```python
from build123d import *

# Parameters (mm, degrees)
F1_DEPTH = 8
F2_R     = 2
F3_R     = 3
F4_R     = 2.5
F5_DEPTH = 8.001
F7_DEPTH = 8.001


with BuildPart() as f1:
    # F0 (on Front) → F1 (new body)
    with BuildSketch(Plane.XZ):
        Polygon((-37.1, 0), (-33.1, 0), (-33.1, 9), (-27.1, 9), (-27.1, 13), (0, 13), (0, 19), (-37.1, 19), align=None)
    extrude(amount=F1_DEPTH)

    # F2
    f2_edges = [f1.edges().sort_by_distance(p)[0] for p in [
        (-27.1, -4, 13),
    ]]
    fillet(f2_edges, radius=F2_R)

    # F3
    f3_edges = [f1.edges().sort_by_distance(p)[0] for p in [
        (-37.1, -4, 19),
    ]]
    fillet(f3_edges, radius=F3_R)

    # F4 (on face) → F5 (cut, through all)
    with BuildSketch(Plane.XZ.offset(8)):
        with Locations((-30.6, 9)):
            Circle(F4_R)
    extrude(amount=-F5_DEPTH, mode=Mode.SUBTRACT)

    # F6 (on face) → F7 (cut, through all)
    with BuildSketch(Plane.XZ.offset(8)):
        with BuildLine():
            Line((-29.1, 19), (-34.1, 19))
            ThreePointArc((-34.1, 19), (-35.8320508076, 18.4494897428), (-36.9284271247, 17))
            Line((-36.9284271247, 17), (-29.1, 17))
            Line((-29.1, 17), (-29.1, 19))
        make_face()
        with BuildLine():
            ThreePointArc((-27.1, 11), (-27.0840593925, 11.252008585), (-27.0364916731, 11.5))
            Line((-27.0364916731, 11.5), (-30.6, 11.5))
            ThreePointArc((-30.6, 11.5), (-28.832233047, 10.767766953), (-28.1, 9))
            Line((-28.1, 9), (-27.1, 9))
            Line((-27.1, 9), (-27.1, 11))
        make_face()
    extrude(amount=-F7_DEPTH, mode=Mode.SUBTRACT)

    # F8: F1 across plane


with BuildPart() as f1_1:
    add(f1.part)
    add(f1.part.mirror(Plane.YZ))


solid = f1_1.part
```
Input: part model. Units: mm. Frame: model coordinates. A direction names the side the tool comes from. Coordinates: 2 decimals unless noted, no trailing zeros. Loops run counter-clockwise (first coordinate to the right, second up) from the corner with the lowest first, then second, coordinate; pieces in that order, holes last.
Q1. Section A-A, the plane z = 6.75. Return the cut outline in (x, y).
Results are:
outline: (-37.1, -8) - (-33.1, -8) - (-33.1, 0) - (-37.1, 0) - close; (33.1, -8) - (37.1, -8) - (37.1, 0) - (33.1, 0) - close
Q2. Section C-C, the plane z = 12.25. Return the cut outline in (x, y), and give its area (3 significant figures).
Results are:
outline: (-37.1, -8) - (-26.66, -8) - (-26.66, 0) - (-37.1, 0) - close; (26.66, -8) - (37.1, -8) - (37.1, 0) - (26.66, 0) - close
area: 167 mm2
Q3. Contact query for flat-ended pins moving along their axis: pin 1 (4 mm diameter, centred on x = -28.5, y = -2, fed in from -Z); pin 2 (2.5 mm diameter, centred on x = -3, y = -3.5, fed in from -Z); pin 3 (4 mm diameter, centred on x = 32, y = -2.5, fed in from +Z). Output: stop coordinate, or through.
Results are:
pin 1: stops at z = 11.5
pin 2: stops at z = 13
pin 3: stops at z = 17
Q4. Section D-D, the plane x = -17. Return the cut outline in (y, z).
Results are:
outline: (-8, 13) - (0, 13) - (0, 19) - (-8, 19) - close
Q5. Mould query, pull axis X, two halves, no side actions, for faces 4 (the flat face through (37.1, -4, 8)), 5 (the cylindrical face through (32.348, -4.056, 10.787)), 6 (the flat face through (33, -4, 17)). Classes: +X half, -X half, draft (parallel to the pull), parting line (faces both ways), or undercut.
Results are:
face 4: +X half
face 5: undercut
face 6: draft
Q6. Line query: line 1 along X through (y, z) = (-3.5, 4.5); line 2 along Z through (x, y) = (-16.5, -0.75); line 3 along X through (y, z) = (-6.5, 12.5). Output: solid intervals per line, ascending.
Results are:
line 1: x = -37.1 to -33.1, 33.1 to 37.1
line 2: z = 13 to 19
line 3: x = -37.1 to -26.42, 26.42 to 37.1
Q7. Set-up query: faces 1 (the flat face through (29.1, -4, 18)), 2 (the flat face through (29, -4, 11.5)), 3 (the flat face through (-29.1, -4, 18)). Return all of +Z, -Z, +X, -X, +Y, -Y with unobstructed straight access to the full face (end or side cutting, diameter ignored); none if empty.
Results are:
face 1: +Z, +X, +Y, -Y
face 2: -Z, +Y, -Y
face 3: +Z, -X, +Y, -Y
Q8. Section B-B, the plane y = -5.75. Return the cut outline in (x, z).
Results are:
outline: (-37.1, 0) - (-33.1, 0) - (-33.1, 9) arc R2.5 cw to (-30.6, 11.5) - (-27.04, 11.5) arc R2 cw to (-25.1, 13) - (25.1, 13) arc R2 cw to (27.04, 11.5) - (30.6, 11.5) arc R2.5 cw to (33.1, 9) - (33.1, 0) - (37.1, 0) - (37.1, 16) arc R3 ccw to (36.93, 17) - (29.1, 17) - (29.1, 19) - (-29.1, 19) - (-29.1, 17) - (-36.93, 17) arc R3 ccw to (-37.1, 16) - close
